```python
from build123d import *

# Parameters (mm, degrees)
SKETCH1_W      = 6.35
SKETCH1_H      = 2.77
EXTRUDE1_DEPTH = 1.27
SKETCH2_W      = 6.35
SKETCH2_H      = 1.27
EXTRUDE2_DEPTH = 4.5
SKETCH3_W      = 4.17
SKETCH3_H      = 4.57
SKETCH3_R      = 0.925
EXTRUDE3_DEPTH = 1.27
FILLET1_R      = 0.81


with BuildPart() as part:
    # Sketch1 → Extrude1 (new body)
    with BuildSketch(Plane.XY):
        Rectangle(SKETCH1_W, SKETCH1_H)
    extrude(amount=EXTRUDE1_DEPTH)

    # Sketch2 → Extrude2 (add)
    with BuildSketch(Plane.XY.offset(1.27)):
        with Locations((0, 0.75)):
            Rectangle(SKETCH2_W, SKETCH2_H)
    extrude(amount=EXTRUDE2_DEPTH)

    # Sketch3 → Extrude3 (add)
    with BuildSketch(Plane.XY.offset(5.77)):
        with Locations((0, -2.17)):
            Rectangle(SKETCH3_W, SKETCH3_H)
        with Locations((0, -0.875)):
            Circle(SKETCH3_R, mode=Mode.SUBTRACT)
    extrude(amount=-EXTRUDE3_DEPTH)

    # Fillet1
    fillet1_edges = [part.edges().sort_by_distance(p)[0] for p in [
        (-2.085, -4.455, 5.135),
        (2.085, -4.455, 5.135),
    ]]
    fillet(fillet1_edges, radius=FILLET1_R)


solid = part.part
```
The model under review builds one solid part; all positions refer to its coordinate system, in mm. A direction names the side the tool comes from. Round coordinates to 2 decimals unless told otherwise and drop trailing zeros. Write each loop counter-clockwise with the first axis right and the second up, starting at its lowest first coordinate (ties: lowest second). Pieces come first, ordered by that corner, then holes.
(1) Machinability: for faces 4 (the flat face through (-2.085, -2, 5)), 5 (the cylindrical face through (-0.2, -1.78, 5.14)), 6 (the flat face through (0, -1, 1.27)), which of the approach directions +Z, -Z, +X, -X, +Y, -Y give a long, thin tool a straight path to every point of the face, cutting with its end or side? Answer none if there is none.
(2) Wall thickness on L1, parallel to Z at x = 1.5, y = -1.05; L2, parallel to Y at x = 0, z = 1.5 (3 decimals); L3, parallel to Z at x = 2, y = -3.9: over which ranges is each line inside the solid? List them lowest first.
(3) We need section B-B on z = 4.75. Give the boundary of the cut face in (x, y) (3 decimals), and give its area (3 significant figures).
(4) Mouldability with a two-part tool opening along Z and no side actions: class faces 1 (the flat face through (0, 0.115, 3)), 2 (the cylindrical face through (-1.854, -4.211, 5.126)), 3 (the flat face through (0, -2, 5.77)) as +Z half, -Z half, draft (parallel to the pull), parting line (faces both ways), or undercut.
(5) We need section C-C on y = -1. Give the boundary of the cut face in (x, z) (3 decimals), and give its area (3 significant figures).
(6) We need section D-D on z = 1.1. Give the boundary of the cut face in (x, y) (3 decimals).
(7) We need section A-A on x = 0. Give the boundary of the cut face in (y, z) (3 decimals).
(8) Insertion check: pin 1 (1.7 mm diameter, centred on x = 0, y = -0.875, fed in from +Z); pin 2 (1.3 mm diameter, centred on x = -1, y = -2.5, fed in from -Z); pin 3 (1 mm diameter, centred on y = -1.5, z = 5.5, fed in from +X) (3 decimals). Each pin has a flat end and moves straight along its axis. Give the tip position at first contact, or say it passes through.
Findings below:
1. face 4: +Z, -X, -Y
1. face 5: +Z
1. face 6: +X, -X, -Y
2. L1: z = 0 to 1.27, 4.5 to 5.77
2. L2: y = 0.115 to 1.385
2. L3: z = 4.5 to 5.77
3. outline: (-3.175, 0.115) - (-2.085, 0.115) - (-2.085, -3.645) arc R0.81 ccw to (-1.275, -4.455) - (1.275, -4.455) arc R0.81 ccw to (2.085, -3.645) - (2.085, 0.115) - (3.175, 0.115) - (3.175, 1.385) - (-3.175, 1.385) - close; hole circle Ø1.85 at (0, -0.875)
3. area: 24.2 mm2
4. face 1: undercut
4. face 2: draft
4. face 3: +Z half
5. outline: (-3.175, 0) - (3.175, 0) - (3.175, 1.27) - (-3.175, 1.27) - close; (-2.085, 4.5) - (-0.917, 4.5) - (-0.917, 5.77) - (-2.085, 5.77) - close; (0.917, 4.5) - (2.085, 4.5) - (2.085, 5.77) - (0.917, 5.77) - close
5. area: 11.0 mm2
6. outline: (-3.175, -1.385) - (3.175, -1.385) - (3.175, 1.385) - (-3.175, 1.385) - close
7. outline: (-4.455, 4.5) - (-1.8, 4.5) - (-1.8, 5.77) - (-4.455, 5.77) - close; (-1.385, 0) - (1.385, 0) - (1.385, 5.77) - (0.05, 5.77) - (0.05, 4.5) - (0.115, 4.5) - (0.115, 1.27) - (-1.385, 1.27) - close
8. pin 1: stops at z = 1.27
8. pin 2: stops at z = 4.5
8. pin 3: stops at x = 2.085
